from build123d import *

# Parameters (mm, degrees)
SKETCH1_R           = 65
SKETCH1_R_2         = 51.5
BOSS_EXTRUDE1_DEPTH = 10
THREAD1_PITCH       = 6
SKETCH10_R          = 1
CUT_EXTRUDE1_DEPTH  = 21


with BuildPart() as part:
    # Sketch1 → Boss-Extrude1 (new body)
    with BuildSketch(Plane.XY):
        Circle(SKETCH1_R)
        Circle(SKETCH1_R_2, mode=Mode.SUBTRACT)
    extrude(amount=BOSS_EXTRUDE1_DEPTH)

    # Thread1: the profile of Thread Profile1 profile screwed along a right-hand helix of 1.5 turns, 14 arcs to a turn; built about Z, then put on its axis
    thread1_z = Axis((0, 0, 0), (0, 0, 1))
    thread1_corners = [(65.0003, -1.9e-08, -0.000173205), (65.0003, -1.9e-08, 5.250173189), (61.75240475, -1.8e-08, 3.374999992), (61.75240475, -1.8e-08, 1.874999992)]
    with BuildLine(mode=Mode.PRIVATE) as thread1_profile:
        Line(thread1_corners[0], thread1_corners[1])
        Line(thread1_corners[1], thread1_corners[2])
        Line(thread1_corners[2], thread1_corners[3])
        Line(thread1_corners[3], thread1_corners[0])
    thread1_cap = Face(thread1_profile.wire())
    thread1_turn_angles = [0, 12.857142857, 25.714285714, 38.571428571, 51.428571429, 64.285714286, 77.142857143, 90, 102.857142857, 115.714285714, 128.571428571, 141.428571429, 154.285714286, 167.142857143, 180, 192.857142857, 205.714285714, 218.571428571, 231.428571429, 244.285714286, 257.142857143, 270, 282.857142857, 295.714285714, 308.571428571, 321.428571429, 334.285714286, 347.142857143, 360]
    thread1_turn_weights = [1, 0.9749279121818236, 1, 0.9749279121818236, 1, 0.9749279121818236, 1, 0.9749279121818236, 1, 0.9749279121818236, 1, 0.9749279121818236, 1, 0.9749279121818236, 1, 0.9749279121818236, 1, 0.9749279121818236, 1, 0.9749279121818236, 1, 0.9749279121818236, 1, 0.9749279121818237, 1, 0.9749279121818236, 1, 0.9749279121818236, 1]
    thread1_turn_rails = [Edge.make_bspline([Vector(p[0], p[1], 0).rotate(thread1_z, thread1_turn_angles[k]) / thread1_turn_weights[k] + Vector(0, 0, p[2] + THREAD1_PITCH * thread1_turn_angles[k] / 360) for k in range(29)], [0, 0, 0, 1, 1, 2, 2, 3, 3, 4, 4, 5, 5, 6, 6, 7, 7, 8, 8, 9, 9, 10, 10, 11, 11, 12, 12, 13, 13, 14, 14, 14], 2, thread1_turn_weights) for p in thread1_corners]
    thread1_turn_sides = [Face.make_surface_from_curves(thread1_turn_rails[p[0]], thread1_turn_rails[p[1]]) for p in [(0, 1), (1, 2), (2, 3), (3, 0)]]
    thread1_last_angles = [360, 372.857142857, 385.714285714, 398.571428571, 411.428571429, 424.285714286, 437.142857143, 450, 462.857142857, 475.714285714, 488.571428571, 501.428571429, 514.285714286, 527.142857143, 540]
    thread1_last_weights = [1, 0.9749279121818236, 1, 0.9749279121818236, 1, 0.9749279121818237, 1, 0.9749279121818235, 1, 0.9749279121818237, 1, 0.9749279121818237, 1, 0.9749279121818235, 1]
    thread1_last_rails = [Edge.make_bspline([Vector(p[0], p[1], 0).rotate(thread1_z, thread1_last_angles[k]) / thread1_last_weights[k] + Vector(0, 0, p[2] + THREAD1_PITCH * thread1_last_angles[k] / 360) for k in range(15)], [0, 0, 0, 1, 1, 2, 2, 3, 3, 4, 4, 5, 5, 6, 6, 7, 7, 7], 2, thread1_last_weights) for p in thread1_corners]
    thread1_last_sides = [Face.make_surface_from_curves(thread1_last_rails[p[0]], thread1_last_rails[p[1]]) for p in [(0, 1), (1, 2), (2, 3), (3, 0)]]
    thread1 = Plane(origin=(0, 0, 9), x_dir=(-0.999390827, 0.034899497, 0), z_dir=(0, 0, -1)) * Solid(Shell([*thread1_turn_sides, *thread1_last_sides, thread1_cap, thread1_cap.rotate(thread1_z, 540).moved(Location((0, 0, THREAD1_PITCH * 540 / 360)))]))
    add(thread1, mode=Mode.SUBTRACT)

    # Sketch10 → Cut-Extrude1 (cut)
    with BuildSketch(Plane(origin=(0, 0, 0), x_dir=(0.9993908270190958, -0.03489949670250096, 0), z_dir=(0.03489949670250096, 0.9993908270190958, 0))):
        with Locations(Location((-63.387356221, -6.373965218, 0), (0, 0, 180))):
            Circle(SKETCH10_R)
    extrude(amount=-CUT_EXTRUDE1_DEPTH, mode=Mode.SUBTRACT)


solid = part.part
Geometry check sheet. Reference: the model listing, model coordinates, mm. Give positions to 0.01 mm unless a question says otherwise; leave off trailing zeros.
1. Depth check by flat-ended pin: pin 1 (3 mm diameter, centred on y = -5.5, z = 5.5, fed in from +X); pin 2 (1.5 mm diameter, centred on x = 13, z = 6.5, fed in from -Y); pin 3 (2 mm diameter, centred on y = 16.5, z = 2, fed in from -X). Enter the tip coordinate at first touch or a pass-through.
Completed:
pin 1: stops at x = 64.87
pin 2: stops at y = -63.84
pin 3: stops at x = -63.03
2. Scan lines: line 1 (Y direction, x = 0, z = 3.25); line 2 (Y direction, x = 35.5, z = 4); line 3 (X direction, y = -16, z = 6.25). Record each from-to range of solid material in increasing order.
Completed:
line 1: y = -62.78 to -51.5, 51.5 to 63.33
line 2: y = -52.15 to -37.31, 37.31 to 50.53
line 3: x = -62.99 to -48.95, 48.95 to 63
3. Sectioned sample at A-A (y = -5). State how many separate pieces and enclosed holes the cut face has, then the cut area to 3 significant figures.
Completed:
separate pieces: 2
enclosed holes: 1
area: 250 mm2
